Design review of the part shown in the three views and the two pictorial views. Dimensions are in mm from the part's minimum x, y and z. A direction names the side the tool comes from. Round coordinates to 2 decimals unless told otherwise and drop trailing zeros. Order: outer loops, then holes, each group sorted by start corner. A loop starts at its lowest first (then second) coordinate and runs counter-clockwise, first axis right, second up.
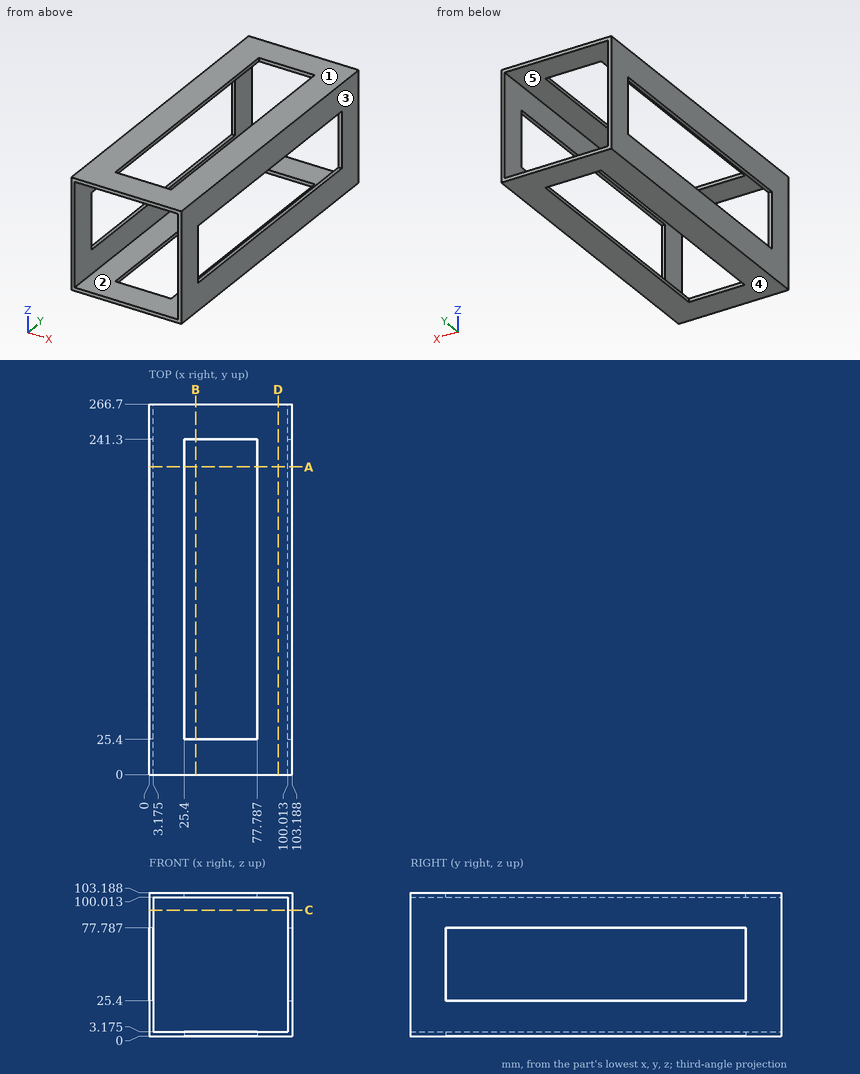
(1) For the marked faces 4 and 5, list the 3-axis set-ups (+Z, -Z, +X, -X, +Y, -Y) from which the entire face can be reached by the end or side of a thin tool; tool diameter is ignored.
Data:
face 4: -Z, +X, -X, +Y, -Y
face 5: +Y, -Y
(2) Consider section B-B (x = 33.5). Write out the cut boundary in (y, z) (1 decimal).
Data:
outline: (0, 0) - (25.4, 0) - (25.4, 3.2) - (0, 3.2) - close; (0, 100) - (25.4, 100) - (25.4, 103.2) - (0, 103.2) - close; (241.3, 0) - (266.7, 0) - (266.7, 3.2) - (241.3, 3.2) - close; (241.3, 100) - (266.7, 100) - (266.7, 103.2) - (241.3, 103.2) - close
(3) Draft analysis for pull direction Z (two halves, no side actions). For the marked faces 1, 2 and 3, state which applies: pulls with the +Z half, pulls with the -Z half, needs draft (parallel to the pull), parting line crosses it, or undercut.
Data:
face 1: pulls with the +Z half
face 2: undercut
face 3: needs draft
(4) To check wall thickness, follow probe 1 along Z at (x, y) = (81.5, 142) (1 decimal). State the ranges of the line that lie inside material, in increasing order.
Data:
probe 1: z = 0 to 3.2, 100 to 103.2
(5) Consider section C-C (z = 90.5). Write out the cut boundary in (x, y) (1 decimal), and give its area (3 significant figures).
Data:
outline: (0, 0) - (3.2, 0) - (3.2, 266.7) - (0, 266.7) - close; (100, 0) - (103.2, 0) - (103.2, 266.7) - (100, 266.7) - close
area: 1,690 mm2
(6) Consider section D-D (x = 93). Write out the cut boundary in (y, z) (1 decimal).
Data:
outline: (0, 0) - (266.7, 0) - (266.7, 3.2) - (0, 3.2) - close; (0, 100) - (266.7, 100) - (266.7, 103.2) - (0, 103.2) - close
(7) Insertion check: pin 1 (2.5 mm diameter, centred on x = 2, z = 40, fed in from -Y). The pin has a flat end and moves straight along its axis. Give the tip position at first contact, or say it passes through.
Data:
pin 1: stops at y = 0
(8) Consider section A-A (y = 221.5). Write out the cut boundary in (x, z) (1 decimal).
Data:
outline: (0, 0) - (25.4, 0) - (25.4, 3.2) - (3.2, 3.2) - (3.2, 25.4) - (0, 25.4) - close; (0, 77.8) - (3.2, 77.8) - (3.2, 100) - (25.4, 100) - (25.4, 103.2) - (0, 103.2) - close; (77.8, 0) - (103.2, 0) - (103.2, 25.4) - (100, 25.4) - (100, 3.2) - (77.8, 3.2) - close; (77.8, 100) - (100, 100) - (100, 77.8) - (103.2, 77.8) - (103.2, 103.2) - (77.8, 103.2) - close
